The listing builds one solid part. Answer for the finished solid, in the listing's coordinates (mm). Give positions to 0.01 mm unless a question says otherwise; leave off trailing zeros. Write each loop counter-clockwise with the first axis right and the second up, starting at its lowest first coordinate (ties: lowest second). Pieces come first, ordered by that corner, then holes. Notation, with made-up numbers: (-28, -2.75) - (0, -2.75) arc R28 ccw to (0, 35.25) - close; hole circle Ø8 at (2.5, -24.5). An arc over 180 degrees is marked (long way). Use a Markdown table: item, result. Add a question column.
Autodesk Inventor part; units mm, degrees
ref_plane "YZ Plane" through (0, 0, 0) normal (1, 0, 0) x (0, 1, 0)
ref_plane "XZ Plane" through (0, 0, 0) normal (0, 1, 0) x (-1, 0, 0)
ref_plane "XY Plane" through (0, 0, 0) normal (0, 0, 1) x (1, 0, 0)
sketch "Sketch2" plane through (0, 0, 0) normal (0, 0, 1) x (1, 0, 0)
  line L0 (-22.1612, -7.9741) -> (-70.1612, -7.9741)
  line L1 (-70.1612, -7.9741) -> (-70.1612, 34.0259)
  line L2 (-70.1612, 34.0259) -> (-22.1612, 34.0259)
  line L3 (-22.1612, 34.0259) -> (-22.1612, -7.9741)
  line L4 (-70.1612, -7.9741) -> (-70.1612, -3.9741)
  line L5 (-70.1612, -3.9741) -> (-60.1612, -3.9741)
  line L6 (-22.1612, -7.9741) -> (-22.1612, -3.9741)
  line L7 (-22.1612, -3.9741) -> (-26.1612, -3.9741)
  circle A0 centre (-60.1612, -3.9741) radius 1.5
  circle A1 centre (-26.1612, -3.9741) radius 1.5
  point P0 (0, 0)
  dimension "d0" = 48
  dimension "d1" = 42
  dimension "d2" = 4
  dimension "d3" = 10
  dimension "d4" = 4
  dimension "d5" = 4
  dimension "d6" = 3
  dimension "d7" = 3
extrude "Extrusion1" add sketch "Sketch2" along normal blind 2
properties part number "driver kort"
1. For a pull along Y with two mould halves and no side action, classify faces 1 (the flat face through (-46, 34.026, 1)), 2 (the flat face through (-46, 13, 0)), 3 (the cylindrical face through (-61.35, -3.06, 0.99)) as released by +Y, released by -Y, zero draft, split by the parting line, or undercut.
2. The part is cut by section A-A (x = -26.5). Give the vertices of the cut face in (y, z).
3. Given P1, Ø1.8, axis at x = -26.16, y = -3.97, coming from the -Z side, flat-ended and moving along its own axis, determine where the tip first touches the part or whether it passes through.
4. Consider L1, parallel to X at y = -3.5, z = 1.2; L2, parallel to X at y = -5, z = 1.25; L3, parallel to Y at x = -27.5, z = 0.9. Determine where each line is inside the solid, lowest interval first. Write a range as [from, to].
Check values:
| question | item | result |
|---|---|---|
| 1 | face 1 | released by +Y |
| 1 | face 2 | zero draft |
| 1 | face 3 | undercut |
| 2 | outline | (-7.97, 0) - (-5.44, 0) - (-5.44, 2) - (-7.97, 2) - close; (-2.51, 0) - (34.03, 0) - (34.03, 2) - (-2.51, 2) - close |
| 3 | P1 | passes through |
| 4 | L1 | x = [-70.16, -61.58], [-58.74, -27.58], [-24.74, -22.16] |
| 4 | L2 | x = [-70.16, -61.26], [-59.07, -27.26], [-25.07, -22.16] |
| 4 | L3 | y = [-7.97, -4.65], [-3.3, 34.03] |
